Work out the finished part from the listing and answer in its coordinate system (mm). A direction names the side the tool comes from. Round coordinates to 2 decimals unless told otherwise and drop trailing zeros. Loops run counter-clockwise (first coordinate to the right, second up) from the corner with the lowest first, then second, coordinate; pieces in that order, holes last. Notation, with made-up numbers: (-39.5, -25) -> (-16.5, -25) arc R9 cw to (-16.5, -18) -> close; hole circle Ø3 at (-5, 39.5). An arc over 180 degrees is marked (long way). Use one line per item in the form item = value.
Autodesk Inventor part; units mm, degrees
ref_plane "YZ Plane" through (0, 0, 0) normal (1, 0, 0) x (0, 1, 0)
ref_plane "XZ Plane" through (0, 0, 0) normal (0, 1, 0) x (-1, 0, 0)
ref_plane "XY Plane" through (0, 0, 0) normal (0, 0, 1) x (1, 0, 0)
sketch "Szkic1" plane through (0, 0, 0) normal (0, 0, 1) x (1, 0, 0)
  line L0 (-89.8533, 62.242) -> (466.1467, 62.242)
  line L1 (466.1467, 62.242) -> (466.1467, 0.242)
  line L2 (466.1467, 0.242) -> (-89.8533, 0.242)
  line L3 (-89.8533, 0.242) -> (-89.8533, 62.242)
  line L4 (75.48, 62.242) -> (105.48, 62.242)
  line L5 (105.48, 62.242) -> (105.48, 90.242)
  line L6 (105.48, 90.242) -> (75.48, 90.242)
  line L7 (75.48, 90.242) -> (75.48, 62.242)
  line L8 (270.8133, 62.242) -> (300.8133, 62.242)
  line L9 (300.8133, 62.242) -> (300.8133, 90.242)
  line L10 (300.8133, 90.242) -> (270.8133, 90.242)
  line L11 (270.8133, 90.242) -> (270.8133, 62.242)
  arc A0 (403.6467, 13.242) -> (407.6467, 17.242) centre (403.6467, 17.242) ccw
  line L12 (407.6467, 17.242) -> (407.6467, 37.242)
  arc A1 (407.6467, 37.242) -> (403.6467, 41.242) centre (403.6467, 37.242) ccw
  line L13 (388.647, 36.242) -> (393.647, 41.242)
  line L14 (388.647, 36.242) -> (388.647, 18.242)
  line L15 (393.647, 13.242) -> (388.647, 18.242)
  line L16 (393.647, 41.242) -> (403.6467, 41.242)
  line L17 (393.647, 13.242) -> (403.6467, 13.242)
  line L18 (393.4399, 41.742) -> (388.147, 36.4491)
  line L19 (388.147, 36.4491) -> (388.147, 18.0348)
  line L20 (388.147, 18.0348) -> (393.4399, 12.742)
  line L21 (393.4399, 12.742) -> (403.6467, 12.742)
  arc A2 (403.6467, 12.742) -> (408.1467, 17.242) centre (403.6467, 17.242) ccw
  line L22 (408.1467, 17.242) -> (408.1467, 37.242)
  arc A3 (408.1467, 37.242) -> (403.6467, 41.742) centre (403.6467, 37.242) ccw
  line L23 (403.6467, 41.742) -> (393.4399, 41.742)
  circle A4 centre (398.6468, 46.742) radius 1.5
  circle A5 centre (398.6467, 7.742) radius 1.5
  line L24 (346.447, 43.242) -> (368.147, 43.242)
  line L25 (368.147, 43.242) -> (368.147, 15.242)
  line L26 (368.147, 15.242) -> (346.447, 15.242)
  line L27 (346.447, 15.242) -> (346.447, 43.242)
  line L28 (276.447, 36.242) -> (292.947, 36.242)
  line L29 (292.947, 36.242) -> (292.947, 22.242)
  line L30 (292.947, 22.242) -> (276.447, 22.242)
  line L31 (276.447, 22.242) -> (276.447, 36.242)
  line L32 (242.947, 36.542) -> (256.447, 36.542)
  line L33 (256.447, 36.542) -> (256.447, 21.942)
  line L34 (256.447, 21.942) -> (242.947, 21.942)
  line L35 (242.947, 21.942) -> (242.947, 36.542)
  line L36 (312.947, 38.742) -> (326.447, 38.742)
  line L37 (326.447, 38.742) -> (326.447, 19.742)
  line L38 (326.447, 19.742) -> (312.947, 19.742)
  line L39 (312.947, 19.742) -> (312.947, 38.742)
  point P0 (90.48, 75.242)
  point P1 (285.8133, 75.242)
  point P2 (-76.3533, 47.242)
  point P3 (452.6467, 47.242)
  point P4 (-76.3533, 15.242)
  point P5 (452.6467, 15.242)
  dimension "d0" = 556
  dimension "d1" = 62
  dimension "d2" = 30
  dimension "d3" = 28
  dimension "d4" = 30
  dimension "d5" = 28
  dimension "d6" = 165.3333
  dimension "d10" = 165.3333
  dimension "d12" = 15
  dimension "d13" = 15
  dimension "d14" = 15
  dimension "d15" = 15
  dimension "d16" = 13.5
  dimension "d17" = 13.5
  dimension "d18" = 15
  dimension "d19" = 15
  dimension "d27" = 13.5
  dimension "d28" = 13.5
  dimension "d29" = 15
  dimension "d30" = 15
  dimension "d42" = 18.9997
  dimension "d43" = 58.5
  dimension "d44" = 28
  dimension "d45" = 21
  dimension "d46" = 14.9997
  dimension "d47" = 4
  dimension "d48" = 4
  dimension "d49" = 14.9997
  dimension "d50" = 5
  dimension "d51" = 5
  dimension "d54" = 0.5
  dimension "d55" = 5.5
  dimension "d56" = 5.5
  dimension "d57" = 8.9999
  dimension "d58" = 9
  dimension "d59" = 3
  dimension "d60" = 3
  dimension "d61" = 10.2068
  dimension "d62" = 9.9997
  dimension "d63" = 9.9997
  dimension "d64" = 10.2068
  dimension "d65" = 28
  dimension "d66" = 21.7
  dimension "d69" = 16.5
  dimension "d71" = 14
  dimension "d72" = 14.6
  dimension "d73" = 13.5
  dimension "d74" = 19
  dimension "d75" = 13.5
  dimension "d76" = 19
  dimension "d77" = 23.5
  dimension "d78" = 26
  dimension "d79" = 25.7
  dimension "d80" = 20
  dimension "d81" = 20
  dimension "d82" = 20
  dimension "d83" = 20
extrude "Wyciągnięcie proste1" add sketch "Szkic1" along normal blind 2 contours L0 L1 L2 L3 | L7 L6 L5 L0 | L11 L10 L9 L0 | L17 L15 L14 L13 L16 A1 L12 A0 | L23 A3 L22 A2 L21 L20 L19 L18 | A4 | A5 | L24 L25 L26 L27 | L28 L29 L30 L31 | L32 L33 L34 L35 | L36 L37 L38 L39
fillet "Zaokrąglenie1" radius 10 8 edges at (75.48, 62.242, 1) (75.48, 90.242, 1) (105.48, 90.242, 1) (105.48, 62.242, 1) (270.8133, 62.242, 1) (270.8133, 90.242, 1) (300.8133, 90.242, 1) (300.8133, 62.242, 1)
hole "Otwór1" at (90.48, 75.242, 0) at (285.8133, 75.242, 0) at (-76.3533, 47.242, 0) at (452.6467, 47.242, 0) at (-76.3533, 15.242, 0) at (452.6467, 15.242, 0) direction (0, 0, 1) diameter 4 end through all
extrude "Wyciągnięcie proste2" cut sketch "Szkic1" along normal through all contours L17 L15 L14 L13 L16 A1 L12 A0 | L23 A3 L22 A2 L21 L20 L19 L18 | A4 | A5 | L24 L25 L26 L27 | L28 L29 L30 L31 | L32 L33 L34 L35 | L36 L37 L38 L39
equation "\"d6\" = -0.333333 * d4 + 0.333333 * d0 - 0.333333 * d2"
equation "\"d10\" = d6"
properties part number "LC_ALU_2mm_Back_Plate"
(1) For faces 4 (the cylindrical face through (267.806, 65.094, 1.014)), 5 (the cylindrical face through (72.47, 65.09, 1.01)), determine the directions among +Z, -Z, +X, -X, +Y, -Y from which every point of the face is accessible in a straight line to the end or side of a thin tool.
Completed:
face_4 = +Z, -Z, +Y
face_5 = +Z, -Z, -X, +Y
(2) Find section B-B, the plane z = 0.85. State how many separate pieces and enclosed holes the cut face has, then the cut area to 3 significant figures.
Completed:
separate_pieces = 1
enclosed_holes = 13
area = 34,200 mm2
(3) Given P1, Ø3.5, axis at x = 452.65, y = 15.24, coming from the -Z side; P2, Ø1, axis at x = 184, z = 0.5, coming from the +Y side; P3, Ø12, axis at x = 91.5, y = 53, coming from the -Z side; P4, Ø0.6, axis at y = 75, z = 1.5, coming from the +X side, each flat-ended and moving along its own axis, determine where each tip first touches the part or whether it passes through.
Completed:
P1 = through
P2 = 62.24
P3 = 0
P4 = 300.81
(4) For a pull along X with two mould halves and no side action, classify faces 1 (the cylindrical face through (297.962, 87.235, 1.014)), 2 (the cylindrical face through (78.487, 87.39, 1.014)), 3 (the cylindrical face through (102.628, 87.235, 1.014)) as +X half, -X half, draft (parallel to the pull), parting line (faces both ways), or undercut.
Completed:
face_1 = +X half
face_2 = -X half
face_3 = undercut
(5) Find section A-A, the plane x = 152.5. Write down the section's boundary in (y, z).
Completed:
outline = (0.24, 0) -> (62.24, 0) -> (62.24, 2) -> (0.24, 2) -> close
(6) Consider L1, parallel to Y at x = 90.48, z = 1.4; L2, parallel to X at y = 17, z = 0.35; L3, parallel to X at y = 38, z = 0.75. Determine where each line is inside the solid, lowest interval first.
Completed:
L1 = 0.24 to 73.24, 77.24 to 90.24
L2 = -89.85 to -77.31, -75.4 to 346.45, 368.15 to 389.18, 408.14 to 451.69, 453.6 to 466.15
L3 = -89.85 to 312.95, 326.45 to 346.45, 368.15 to 389.7, 408.08 to 466.15
